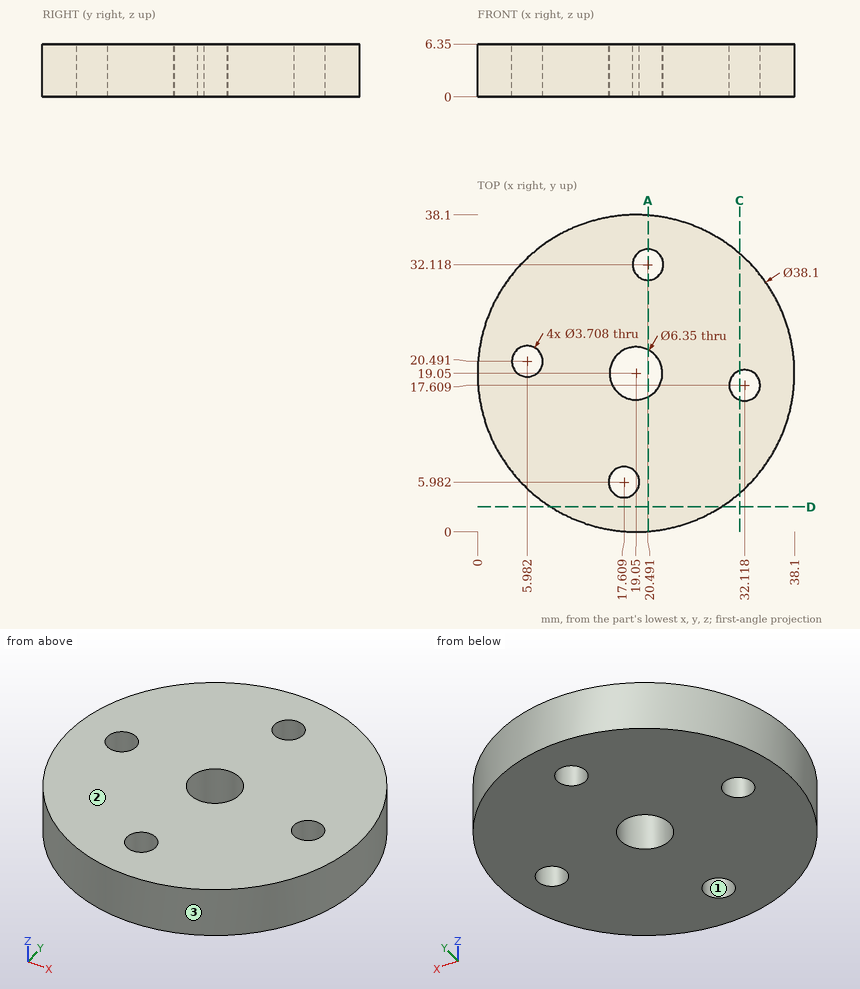
Study the drawing (mm; zero at the part's minimum x, y, z) and answer. Coordinates: 2 decimals unless noted, no trailing zeros. Write each loop counter-clockwise with the first axis right and the second up, starting at its lowest first coordinate (ties: lowest second). Pieces come first, ordered by that corner, then holes.
Q1. Given P1, Ø3, axis at x = 30, z = 5.5, coming from the -Y side, flat-ended and moving along its own axis, determine where the tip first touches the part or whether it passes through.
Returned:
P1: stops at y = 2.51
Q2. The mould has two halves that part along X. Classify the marked faces 1, 2 and 3: released by +X, released by -X, zero draft, split by the parting line, or undercut.
Returned:
face 1: undercut
face 2: zero draft
face 3: split by the parting line
Q3. Find the intervals of material crossed by line 1 along X through (y, z) = (20, 2.5) (1 decimal); line 2 along Y through (x, z) = (5.5, 5); line 3 along Y through (x, z) = (21, 1.25) (1 decimal), in increasing order.
Returned:
line 1: x = 0 to 4.2, 7.8 to 16, 22.1 to 38.1
line 2: y = 5.66 to 18.7, 22.28 to 32.44
line 3: y = 0.1 to 16.5, 21.6 to 30.3, 33.9 to 38
Q4. Section D-D, the plane y = 3 is taken. Write down the section's boundary in (x, z), then the cut area to 3 significant figures.
Returned:
outline: (8.79, 0) - (29.31, 0) - (29.31, 6.35) - (8.79, 6.35) - close
area: 130 mm2
Q5. Section A-A, the plane x = 20.5 is taken. Give the number of separate pieces and of enclosed holes in the cut face, then the cut area to 3 significant figures.
Returned:
separate pieces: 3
enclosed holes: 0
area: 182 mm2
Q6. Section C-C, the plane x = 31.5 is taken. Write down the section's boundary in (y, z).
Returned:
outline: (4.63, 0) - (15.86, 0) - (15.86, 6.35) - (4.63, 6.35) - close; (19.36, 0) - (33.47, 0) - (33.47, 6.35) - (19.36, 6.35) - close
